from build123d import *

# Parameters (mm, degrees)
SPLINE_HUB_ENVELOPE_START             = 12.2
SPLINE_HUB_ENVELOPE_PROFILE_R         = 5.5
SPLINE_HUB_ENVELOPE_PROFILE_R_2       = 2.75
SPLINE_HUB_ENVELOPE_DEPTH             = 2
DISC_D20_PCD14_TAP_DRILLS_START       = 14.2
DISC_D20_PCD14_TAP_DRILLS_PROFILE_R   = 10
DISC_D20_PCD14_TAP_DRILLS_PROFILE_R_2 = 2.75
DISC_D20_PCD14_TAP_DRILLS_PROFILE_R_3 = 1.25
DISC_D20_PCD14_TAP_DRILLS_DEPTH       = 2.5


with BuildPart() as part:
    # Spline_hub_envelope_Profile → Spline_hub_envelope (new body)
    with BuildSketch(Plane.XY.offset(SPLINE_HUB_ENVELOPE_START)):
        with Locations((12.5, 0)):
            Circle(SPLINE_HUB_ENVELOPE_PROFILE_R)
        with Locations((12.5, 0)):
            Circle(SPLINE_HUB_ENVELOPE_PROFILE_R_2, mode=Mode.SUBTRACT)
    extrude(amount=SPLINE_HUB_ENVELOPE_DEPTH)

    # Disc_D20_PCD14_tap_drills_Profile → Disc_D20_PCD14_tap_drills (add)
    with BuildSketch(Plane.XY.offset(DISC_D20_PCD14_TAP_DRILLS_START)):
        with Locations((12.5, 0)):
            Circle(DISC_D20_PCD14_TAP_DRILLS_PROFILE_R)
        with Locations((12.5, 0)):
            Circle(DISC_D20_PCD14_TAP_DRILLS_PROFILE_R_2, mode=Mode.SUBTRACT)
        with Locations((19.5, 0)):
            Circle(DISC_D20_PCD14_TAP_DRILLS_PROFILE_R_3, mode=Mode.SUBTRACT)
        with Locations((5.5, 0)):
            Circle(DISC_D20_PCD14_TAP_DRILLS_PROFILE_R_3, mode=Mode.SUBTRACT)
        with Locations((12.5, 7)):
            Circle(DISC_D20_PCD14_TAP_DRILLS_PROFILE_R_3, mode=Mode.SUBTRACT)
        with Locations((12.5, -7)):
            Circle(DISC_D20_PCD14_TAP_DRILLS_PROFILE_R_3, mode=Mode.SUBTRACT)
    extrude(amount=DISC_D20_PCD14_TAP_DRILLS_DEPTH)


solid = part.part
Can you work these out from the model? Positions are in its coordinate system, mm. A direction names the side the tool comes from. Round coordinates to 2 decimals unless told otherwise and drop trailing zeros. Write each loop counter-clockwise with the first axis right and the second up, starting at its lowest first coordinate (ties: lowest second). Pieces come first, ordered by that corner, then holes. Notation, with made-up numbers: (66, 32.25) - (70, 32.25) arc R19 ccw to (70, 60.25) - close; hole circle Ø6 at (19.5, 50). An arc over 180 degrees is marked (long way). Write each question's results on one line, items separated by ' | '. Start each with the question number.
1) Suppose I cut it at A-A (y = 0). List the corners of the cut face in (x, z) for me.
2) Suppose I cut it at D-D (y = 7.25). List the corners of the cut face in (x, z) for me.
3) Suppose I cut it at B-B (z = 16). List the corners of the cut face in (x, y) for me, and give its area (3 significant figures).
4) For pin 1 Ø5 at (x, y) = (7, -7.5) entering from -Z; pin 2 Ø1.5 at (x, y) = (19.5, 0) entering from -Z, each with a flat end and sliding along its axis, tell me the tip position at first contact or that it passes through.
5) Suppose I cut it at C-C (x = 12.5). List the corners of the cut face in (y, z) for me, and give its area (4 significant figures).
6) Please list where these lines run through material, in increasing order: line 1 (Y direction, x = 12.5, z = 15.15); line 2 (X direction, y = 0.25, z = 15.85); line 3 (Z direction, x = 4, y = -1).
7) Which directions (+Z, -Z, +X, -X, +Y, -Y) give clear straight access to the entire face, cutting with the end or side of a thin tool? Please do faces 1 (the cylindrical face through (4.25, 0.05, 15.43)), 2 (the cylindrical face through (17.58, -2.11, 13.19)).
8) We'd pull the mould along X, two halves only. Please class faces 3 (the cylindrical face through (11.51, 6.24, 15.43)), 4 (the flat face through (14, 3, 12.2)), 5 (the cylindrical face through (22.04, 3, 15.43)): released by +X, released by -X, zero draft, split by the parting line, or undercut.
Here are the results:
1) outline: (2.5, 14.2) - (4.25, 14.2) - (4.25, 16.7) - (2.5, 16.7) - close; (6.75, 14.2) - (7, 14.2) - (7, 12.2) - (9.75, 12.2) - (9.75, 16.7) - (6.75, 16.7) - close; (15.25, 12.2) - (18, 12.2) - (18, 14.2) - (18.25, 14.2) - (18.25, 16.7) - (15.25, 16.7) - close; (20.75, 14.2) - (22.5, 14.2) - (22.5, 16.7) - (20.75, 16.7) - close
2) outline: (5.61, 14.2) - (11.28, 14.2) - (11.28, 16.7) - (5.61, 16.7) - close; (13.72, 14.2) - (19.39, 14.2) - (19.39, 16.7) - (13.72, 16.7) - close
3) outline: circle Ø20 at (12.5, 0); hole circle Ø2.5 at (5.5, 0); hole circle Ø5.5 at (12.5, 0); hole circle Ø2.5 at (12.5, -7); hole circle Ø2.5 at (12.5, 7); hole circle Ø2.5 at (19.5, 0) | area: 271 mm2
4) pin 1: stops at z = 14.2 | pin 2: passes through
5) outline: (-10, 14.2) - (-8.25, 14.2) - (-8.25, 16.7) - (-10, 16.7) - close; (-5.75, 14.2) - (-5.5, 14.2) - (-5.5, 12.2) - (-2.75, 12.2) - (-2.75, 16.7) - (-5.75, 16.7) - close; (2.75, 12.2) - (5.5, 12.2) - (5.5, 14.2) - (5.75, 14.2) - (5.75, 16.7) - (2.75, 16.7) - close; (8.25, 14.2) - (10, 14.2) - (10, 16.7) - (8.25, 16.7) - close | area: 34.75 mm2
6) line 1: y = -10 to -8.25, -5.75 to -2.75, 2.75 to 5.75, 8.25 to 10 | line 2: x = 2.5 to 4.28, 6.72 to 9.76, 15.24 to 18.28, 20.72 to 22.5 | line 3: z = 14.2 to 16.7
7) face 1: +Z, -Z | face 2: -Z
8) face 3: undercut | face 4: zero draft | face 5: split by the parting line
